Read the model definition and answer for the solid it produces. Units are mm, in the model's axes. Coordinates: 2 decimals unless noted, no trailing zeros. Loops run counter-clockwise (first coordinate to the right, second up) from the corner with the lowest first, then second, coordinate; pieces in that order, holes last. Notation, with made-up numbers: M -29.75,-31 L -22.75,-31 A25 ccw -22.75,-6 Z; hole C 44,47.5 d5. An arc over 180 degrees is marked long. Use one line per item in the form item = value. Start each with the question number.
1. The part is cut by section A-A (x = 19). Give the vertices of the cut face in (y, z), plus the area to 3 significant figures.
2. Flat-ended cylindrical pins translate along their axes: pin 1 (7 mm diameter, centred on x = 78.5, y = 3.5, fed in from -Z); pin 2 (1.5 mm diameter, centred on x = 78.5, z = 163.5, fed in from +Y). Find the tip coordinate at first contact, or state that the pin passes through.
3. The part is cut by section B-B (z = 177.5). Give the vertices of the cut face in (x, y).
4. The part is cut by section C-C (y = 20). Give the vertices of the cut face in (x, z).
5. Find the intervals of material crossed by probe 1 along Z at (x, y) = (100, 2); probe 2 along Y at (x, z) = (51.5, 82); probe 3 along Z at (x, y) = (22, 31), in increasing order. Write a range as [from, to].
Autodesk Inventor part; units mm, degrees
ref_plane "YZ Plane" through (0, 0, 0) normal (1, 0, 0) x (0, 1, 0)
ref_plane "XZ Plane" through (0, 0, 0) normal (0, 1, 0) x (-1, 0, 0)
ref_plane "XY Plane" through (0, 0, 0) normal (0, 0, 1) x (1, 0, 0)
sketch "Sketch1" plane through (0, 0, 0) normal (1, 0, 0) x (0, 1, 0)
  line L0 (0, 0) -> (6.35, 0)
  line L1 (6.35, 0) -> (6.35, 254)
  line L2 (6.35, 254) -> (0, 254)
  line L3 (0, 254) -> (0, 0)
  line L4 (0, 0) -> (32.6536, -38.9151)
  line L5 (0, 0) -> (50.8, 0) construction
  line L6 (32.6536, -38.9151) -> (37.518, -34.8334)
  line L7 (37.518, -34.8334) -> (6.35, 0)
  dimension "d0" = 6.35
  dimension "d1" = 254
  dimension "d2" = 50.8
  dimension "d3" = 50
  dimension "d4" = 6.35
extrude "Extrusion1" add sketch "Sketch1" along normal blind 25.4
sketch "Sketch2" plane through (25.4, 0, 0) normal (1, 0, 0) x (0, 0, -1)
  line L0 (-254, 6.35) -> (-254, 0)
  line L1 (-254, 0) -> (0, 0)
  line L2 (-254, 6.35) -> (0, 6.35)
  line L3 (0, 6.35) -> (0, 0)
  line L4 (0, 0) -> (-254, 0)
  line L5 (-254, 0) -> (-254, 6.35)
extrude "Extrusion2" add sketch "Sketch2" along normal blind 152.4
properties part number "Ball Blocker"
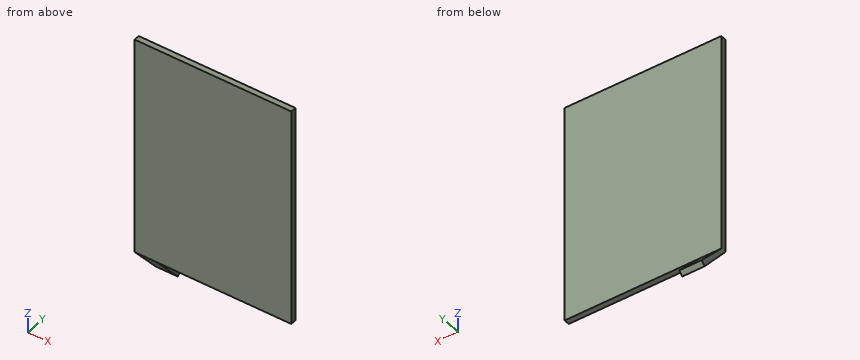
Computed values:
q1.outline = M 0,0 L 32.65,-38.92 L 37.52,-34.83 L 6.35,0 L 6.35,254 L 0,254 Z
q1.area = 1,880 mm²
q2.pin_1 = 0
q2.pin_2 = 6.35
q3.outline = M 0,0 L 177.8,0 L 177.8,6.35 L 0,6.35 Z
q4.outline = M 0,-23.84 L 25.4,-23.84 L 25.4,-15.26 L 0,-15.26 Z
q5.probe_1 = [0, 254]
q5.probe_2 = [0, 6.35]
q5.probe_3 = [-36.94, -27.55]
